Check sheet for the modelled part. Datum: model origin and axes. Units: mm. A direction names the side the tool comes from. Round coordinates to 2 decimals unless told otherwise and drop trailing zeros. Order: outer loops, then holes, each group sorted by start corner. A loop starts at its lowest first (then second) coordinate and runs counter-clockwise, first axis right, second up. Notation, with made-up numbers: (-17, 47.5) -> (-2, 47.5) arc R34 ccw to (-2, 85.5) -> close; hole circle Ø8 at (52, -39.5). An arc over 180 degrees is marked (long way). Answer as CSV lines item,"result". Start each with the question number.
from build123d import *

# Parameters (mm, degrees)
F0_R     = 20
F1_DEPTH = 15
F2_SIZE  = 0.5


with BuildPart() as f1:
    # F0 (on Top) → F1 (new body)
    with BuildSketch(Plane.XY):
        Circle(F0_R)
        with BuildLine():
            ThreePointArc((3.054661, -1.274813), (0, -3.31), (-3.054661, -1.274813))
            ThreePointArc((-3.054661, -1.274813), (-4.1, 0), (-3.054661, 1.274813))
            ThreePointArc((-3.054661, 1.274813), (0, 3.31), (3.054661, 1.274813))
            ThreePointArc((3.054661, 1.274813), (4.1, 0), (3.054661, -1.274813))
        make_face(mode=Mode.SUBTRACT)
    extrude(amount=F1_DEPTH)

    # F2
    f2_edges = [f1.edges().sort_by_distance(p)[0] for p in [
        (-20, 0, 15),
        (-20, 0, 0),
    ]]
    chamfer(f2_edges, length=F2_SIZE)


solid = f1.part
1) Depth check by flat-ended pin: pin 1 Ø1.5 at (y, z) = (-8.5, 11) entering from +X; pin 2 Ø1.5 at (x, z) = (-1.5, 6) entering from -Y. Enter the tip coordinate at first touch or a pass-through.
2) Mould release check, pull along X, two halves, no side actions. Record for faces 1 (the face through (-4.336, -19.524, 7.402)), 2 (the face through (0, -4, 0)), 3 (the face through (-0.05, 3.31, 7.4)), 4 (the face through (-4.1, 0, 7.4)): released by +X, released by -X, zero draft, split by the parting line, or undercut.
3) Section check B-B on y = 0. Record the cut outline in (x, z), then the cut area to 4 significant figures.
4) Material ranges on line 1 along Y through (x, z) = (2, 13.5); line 2 along X through (y, z) = (10, 11.75); line 3 along X through (y, z) = (12, 11.75), recorded low to high.
5) Section check C-C on z = 6. Record the cut outline in (x, y), then the cut area to 3 significant figures.
6) Access from +Z, -Z, +X, -X, +Y, -Y to the whole of each face (thin tool, end or side, straight path). Record for faces 5 (the face through (0, -4, 15)), 6 (the face through (4.1, 0, 7.4)).
7) Section check A-A on x = 0. Record the cut outline in (y, z), then the cut area to 3 significant figures.
Solutions:
1,pin 1,"stops at x = 18.44"
1,pin 2,"stops at y = -19.99"
2,face 1,"split by the parting line"
2,face 2,"zero draft"
2,face 3,"undercut"
2,face 4,"undercut"
3,outline,"(-20, 0.5) -> (-19.5, 0) -> (-4.1, 0) -> (-4.1, 15) -> (-19.5, 15) -> (-20, 14.5) -> close; (4.1, 0) -> (19.5, 0) -> (20, 0.5) -> (20, 14.5) -> (19.5, 15) -> (4.1, 15) -> close"
3,area,"476.5 mm^2"
4,line 1,"y = -19.9 to -2.64, 2.64 to 19.9"
4,line 2,"x = -17.32 to 17.32"
4,line 3,"x = -16 to 16"
5,outline,"circle Ø40 at (0, 0); hole (-3.05, -1.27) arc R3.31 ccw to (3.05, -1.27) arc R1.3 ccw to (3.05, 1.27) arc R3.31 ccw to (-3.05, 1.27) arc R1.3 ccw to start"
5,area,"1,220 mm^2"
6,face 5,"+Z, +X, -X, +Y, -Y"
6,face 6,"+Z, -Z"
7,outline,"(-20, 0.5) -> (-19.5, 0) -> (-3.31, 0) -> (-3.31, 15) -> (-19.5, 15) -> (-20, 14.5) -> close; (3.31, 0) -> (19.5, 0) -> (20, 0.5) -> (20, 14.5) -> (19.5, 15) -> (3.31, 15) -> close"
7,area,"500 mm^2"
